The model under review builds one solid part; all positions refer to its coordinate system, in mm. Face numbers are marked on the shaded views. A direction names the side the tool comes from. Give positions to 0.01 mm unless a question says otherwise; leave off trailing zeros. Loops run counter-clockwise (first coordinate to the right, second up) from the corner with the lowest first, then second, coordinate; pieces in that order, holes last. Notation, with made-up numbers: M 83.25,-12.5 L 92.25,-12.5 A38 ccw 92.25,26.5 Z; hole C -34,85 d11. An arc over 180 degrees is marked long. One line per item, written item: value. Start each with the question number.
Q1. Mouldability with a two-part tool opening along X and no side actions: class the marked faces 1, 2 and 3 as released by +X, released by -X, zero draft, split by the parting line, or undercut.
Q2. We need section D-D on x = -3.5. Write out the cut boundary in (y, z).
Q3. For the marked faces 4 and 5, list the 3-axis set-ups (+Z, -Z, +X, -X, +Y, -Y) from which the entire face can be reached by the end or side of a thin tool; tool diameter is ignored.
Q4. To check wall thickness, follow line 1 along X through (y, z) = (14, 40); line 2 along Z through (x, y) = (26, 0); line 3 along Z through (x, y) = (1, -4). State the ranges of each line that lie inside material, in increasing order. Write a range as from..to.
Q5. We need section B-B on y = 2. Write out the cut boundary in (x, z).
Q6. We need section C-C on y = 9. Write out the cut boundary in (x, z).
Q7. For pin 1 (12 mm diameter, centred on x = -8.5, y = -1, fed in from +Z), flat-tipped, find the tip position at first contact; note if it passes through.
Q8. We need section A-A on z = 7. Write out the cut boundary in (x, y), plus the area to 3 significant figures.
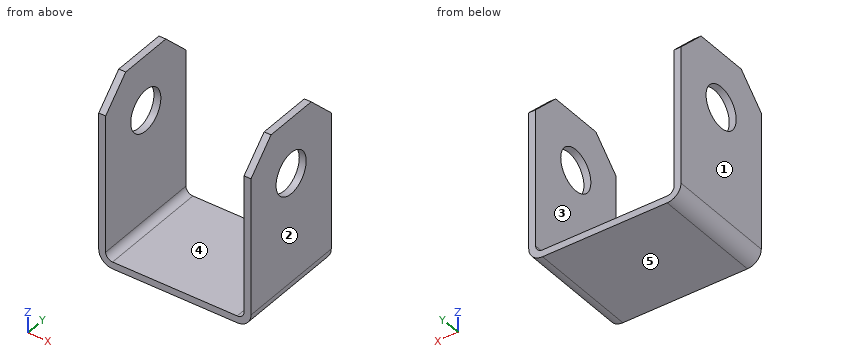
```python
from build123d import *

# Parameters (mm, degrees)
F0_W          = 55
F0_H          = 64.6272003651
F1_DEPTH      = 20
F1_DEPTH_BACK = 20
F2_SIZE       = 10
F3_R          = 5
F4_T          = -2.5
F6_D          = 15


with BuildPart() as f1:
    # F0 (on Front) → F1 (new body, two sides)
    with BuildSketch(Plane.XZ) as f1_sk:
        with Locations((0, 32.3136001825)):
            Rectangle(F0_W, F0_H)
    extrude(amount=F1_DEPTH)
    extrude(f1_sk.sketch, amount=-F1_DEPTH_BACK)

    # F2
    f2_edges = [f1.edges().sort_by_distance(p)[0] for p in [
        (0, -20, 64.6272),
        (0, 20, 64.6272),
    ]]
    chamfer(f2_edges, length=F2_SIZE)

    # F3
    f3_edges = [f1.edges().sort_by_distance(p)[0] for p in [
        (-27.5, 0, 0),
        (27.5, 0, 0),
    ]]
    fillet(f3_edges, radius=F3_R)

    # F4
    f4_openings = [f1.faces().sort_by_distance(p)[0] for p in [
        (0, -20, 27.407493),
        (0, -15, 59.6272),
        (0, 0, 64.6272),
        (0, 15, 59.6272),
        (0, 20, 27.407493),
    ]]
    offset(amount=F4_T, openings=f4_openings)

    # F6 (through all)
    with Locations(Plane(origin=(-27.5, 0, 0), x_dir=(0, -1, 0), z_dir=(-1, 0, 0))):
        with Locations((0, 44.6272003651)):
            Hole(F6_D / 2)


solid = f1.part
```
Solved:
1. face 1: released by -X
1. face 2: released by +X
1. face 3: undercut
2. outline: M -20,0 L 20,0 L 20,2.5 L -20,2.5 Z
3. face 4: +Z, +Y, -Y
3. face 5: -Z, +X, -X, +Y, -Y
4. line 1: -27.5..-25, 25..27.5
4. line 2: 1.43..37.13, 52.13..64.63
4. line 3: 0..2.5
5. outline: M -27.5,5 A5 ccw -22.5,0 L 22.5,0 A5 ccw 27.5,5 L 27.5,37.4 L 25,37.4 L 25,5 A2.5 cw 22.5,2.5 L -22.5,2.5 A2.5 cw -25,5 L -25,37.4 L -27.5,37.4 Z; M -27.5,51.86 L -25,51.86 L -25,64.63 L -27.5,64.63 Z; M 25,51.86 L 27.5,51.86 L 27.5,64.63 L 25,64.63 Z
6. outline: M -27.5,5 A5 ccw -22.5,0 L 22.5,0 A5 ccw 27.5,5 L 27.5,64.63 L 25,64.63 L 25,5 A2.5 cw 22.5,2.5 L -22.5,2.5 A2.5 cw -25,5 L -25,64.63 L -27.5,64.63 Z
7. pin 1: z = 2.5
8. outline: M -27.5,-20 L -25,-20 L -25,20 L -27.5,20 Z; M 25,-20 L 27.5,-20 L 27.5,20 L 25,20 Z
8. area: 200 mm2
